```python
from build123d import *

# Parameters (mm, degrees)
SKETCH1_W           = 147.32
SKETCH1_H           = 63.5
BOSS_EXTRUDE3_DEPTH = 5.08
FILLET4_R           = 12.7
SKETCH4_W           = 121.92
SKETCH4_H           = 63.5
SKETCH4_W_2         = 116.84
SKETCH4_H_2         = 58.42
BOSS_EXTRUDE4_DEPTH = 30.48
SKETCH9_W           = 10.16
SKETCH9_H           = 10.16
BOSS_EXTRUDE5_DEPTH = 5.08
FILLET9_R           = 5.08
SKETCH10_R          = 3.175
CUT_EXTRUDE7_DEPTH  = 163.421034352
FILLET11_R          = 5.08
FILLET12_R          = 7.62
CUT_EXTRUDE8_REACH  = 166.317
SKETCH12_W          = 15.24
SKETCH12_H          = 10.16
FILLET13_R          = 2.54
SKETCH13_W          = 7.62
SKETCH13_H          = 10.16
CUT_EXTRUDE9_DEPTH  = 165.316602935
FILLET14_R          = 2.032
SKETCH11_R          = 3.175
SKETCH11_R_2        = 1.27
BOSS_EXTRUDE7_DEPTH = 5.08
SKETCH15_R          = 1.27
CUT_EXTRUDE10_DEPTH = 2.54
BOSS_EXTRUDE9_START = -2.54
SKETCH16_R          = 3.175
BOSS_EXTRUDE9_DEPTH = 2.54


with BuildPart() as part:
    # Sketch1 → Boss-Extrude3 (new body)
    with BuildSketch(Plane(origin=(0, 0, 0), x_dir=(1, 0, 0), z_dir=(0, 1, 0))):
        with Locations((73.66, 31.75)):
            Rectangle(SKETCH1_W, SKETCH1_H)
    extrude(amount=BOSS_EXTRUDE3_DEPTH)

    # Fillet4
    fillet4_edges = [part.edges().sort_by_distance(p)[0] for p in [
        (0, 2.54, -63.5),
        (147.32, 2.54, -63.5),
        (147.32, 2.54, 0),
        (0, 2.54, 0),
    ]]
    fillet(fillet4_edges, radius=FILLET4_R)

    # Sketch4 → Boss-Extrude4 (add)
    with BuildSketch(Plane(origin=(0, 5.08, 0), x_dir=(1, 0, 0), z_dir=(0, 1, 0))):
        with Locations((73.66, 31.75)):
            Rectangle(SKETCH4_W, SKETCH4_H)
        with Locations((73.66, 31.75)):
            Rectangle(SKETCH4_W_2, SKETCH4_H_2, mode=Mode.SUBTRACT)
    extrude(amount=BOSS_EXTRUDE4_DEPTH)

    # Sketch9 → Boss-Extrude5 (add)
    with BuildSketch(Plane(origin=(0, 5.08, 0), x_dir=(1, 0, 0), z_dir=(0, 1, 0))):
        with Locations((20.32, 55.88)):
            Rectangle(SKETCH9_W, SKETCH9_H)
        with Locations((127, 55.88)):
            Rectangle(SKETCH9_W, SKETCH9_H)
        with Locations((127, 7.62)):
            Rectangle(SKETCH9_W, SKETCH9_H)
        with Locations((20.32, 7.62)):
            Rectangle(SKETCH9_W, SKETCH9_H)
    extrude(amount=BOSS_EXTRUDE5_DEPTH)

    # Fillet9
    fillet9_edges = [part.edges().sort_by_distance(p)[0] for p in [
        (25.4, 7.62, -12.7),
        (25.4, 7.62, -50.8),
        (121.92, 7.62, -50.8),
        (121.92, 7.62, -12.7),
    ]]
    fillet(fillet9_edges, radius=FILLET9_R)

    # Sketch10 → Cut-Extrude7 (cut, through all)
    with BuildSketch(Plane(origin=(0, 10.16, 0), x_dir=(1, 0, 0), z_dir=(0, 1, 0))):
        with Locations(Location((20.32, 55.88, 0), (0, 0, 270))):
            Circle(SKETCH10_R)
        with Locations(Location((127, 55.88, 0), (0, 0, 270))):
            Circle(SKETCH10_R)
        with Locations(Location((20.32, 7.62, 0), (0, 0, 270))):
            Circle(SKETCH10_R)
        with Locations(Location((127, 7.62, 0), (0, 0, 270))):
            Circle(SKETCH10_R)
    extrude(amount=-CUT_EXTRUDE7_DEPTH, mode=Mode.SUBTRACT)

    # Fillet11
    fillet11_edges = [part.edges().sort_by_distance(p)[0] for p in [
        (15.24, 22.86, -2.54),
        (132.08, 22.86, -2.54),
        (132.08, 22.86, -60.96),
        (15.24, 22.86, -60.96),
    ]]
    fillet(fillet11_edges, radius=FILLET11_R)

    # Fillet12
    fillet12_edges = [part.edges().sort_by_distance(p)[0] for p in [
        (12.7, 20.32, -63.5),
        (12.7, 20.32, 0),
        (134.62, 20.32, 0),
        (134.62, 20.32, -63.5),
    ]]
    fillet(fillet12_edges, radius=FILLET12_R)

    # Sketch12 → Cut-Extrude8 (cut, up to next)
    with BuildSketch(Plane.XY, mode=Mode.PRIVATE) as cut_extrude8_sk1:
        with Locations((105.41, 24.257)):
            Rectangle(SKETCH12_W, SKETCH12_H)
    cut_extrude8_tool1 = extrude(cut_extrude8_sk1.sketch, amount=-CUT_EXTRUDE8_REACH, mode=Mode.PRIVATE) & part.part
    add(cut_extrude8_tool1.solids().sort_by_distance((105.41, 24.257, 0))[0], mode=Mode.SUBTRACT)

    # Fillet13
    fillet13_edges = [part.edges().sort_by_distance(p)[0] for p in [
        (97.79, 19.177, -1.27),
        (97.79, 29.337, -1.27),
        (113.03, 29.337, -1.27),
        (113.03, 19.177, -1.27),
    ]]
    fillet(fillet13_edges, radius=FILLET13_R)

    # Sketch13 → Cut-Extrude9 (cut, through all)
    with BuildSketch(Plane.XY):
        with Locations((30.48, 15.24)):
            Rectangle(SKETCH13_W, SKETCH13_H)
        with Locations((53.34, 15.24)):
            Rectangle(SKETCH13_W, SKETCH13_H)
    extrude(amount=-CUT_EXTRUDE9_DEPTH, mode=Mode.SUBTRACT)

    # Fillet14
    fillet14_edges = [part.edges().sort_by_distance(p)[0] for p in [
        (26.67, 10.16, -1.27),
        (26.67, 20.32, -1.27),
        (34.29, 20.32, -1.27),
        (34.29, 10.16, -1.27),
        (26.67, 10.16, -62.23),
        (26.67, 20.32, -62.23),
        (34.29, 20.32, -62.23),
        (34.29, 10.16, -62.23),
        (49.53, 10.16, -1.27),
        (49.53, 20.32, -1.27),
        (57.15, 20.32, -1.27),
        (57.15, 10.16, -1.27),
        (49.53, 10.16, -62.23),
        (49.53, 20.32, -62.23),
        (57.15, 20.32, -62.23),
        (57.15, 10.16, -62.23),
    ]]
    fillet(fillet14_edges, radius=FILLET14_R)

    # Sketch11 → Boss-Extrude7 (add)
    # profile 1 of 4: a face of its own
    with BuildSketch(Plane(origin=(0, 10.16, 0), x_dir=(1, 0, 0), z_dir=(0, 1, 0))):
        with Locations(Location((20.32, 55.88, 0), (0, 0, 270))):
            Circle(SKETCH11_R)
        with Locations(Location((20.32, 55.88, 0), (0, 0, 270))):
            Circle(SKETCH11_R_2, mode=Mode.SUBTRACT)
    # profile 2 of 4: a face of its own
    with BuildSketch(Plane(origin=(0, 10.16, 0), x_dir=(1, 0, 0), z_dir=(0, 1, 0))):
        with Locations(Location((127, 55.88, 0), (0, 0, 270))):
            Circle(SKETCH11_R)
        with Locations(Location((127, 55.88, 0), (0, 0, 270))):
            Circle(SKETCH11_R_2, mode=Mode.SUBTRACT)
    # profile 3 of 4: a face of its own
    with BuildSketch(Plane(origin=(0, 10.16, 0), x_dir=(1, 0, 0), z_dir=(0, 1, 0))):
        with Locations(Location((20.32, 7.62, 0), (0, 0, 270))):
            Circle(SKETCH11_R)
        with Locations(Location((20.32, 7.62, 0), (0, 0, 270))):
            Circle(SKETCH11_R_2, mode=Mode.SUBTRACT)
    # profile 4 of 4: a face of its own
    with BuildSketch(Plane(origin=(0, 10.16, 0), x_dir=(1, 0, 0), z_dir=(0, 1, 0))):
        with Locations(Location((127, 7.62, 0), (0, 0, 270))):
            Circle(SKETCH11_R)
        with Locations(Location((127, 7.62, 0), (0, 0, 270))):
            Circle(SKETCH11_R_2, mode=Mode.SUBTRACT)
    extrude(amount=-BOSS_EXTRUDE7_DEPTH)

    # Sketch15 → Cut-Extrude10 (cut)
    with BuildSketch(Plane(origin=(0, 5.08, 0), x_dir=(1, 0, 0), z_dir=(0, 1, 0))):
        with Locations(Location((6.35, 50.8, 0), (0, 0, 270))):
            Circle(SKETCH15_R)
        with Locations(Location((6.35, 12.7, 0), (0, 0, 270))):
            Circle(SKETCH15_R)
        with Locations(Location((140.97, 12.7, 0), (0, 0, 90))):
            Circle(SKETCH15_R)
        with Locations(Location((140.97, 50.8, 0), (0, 0, 90))):
            Circle(SKETCH15_R)
    extrude(amount=-CUT_EXTRUDE10_DEPTH, mode=Mode.SUBTRACT)

    # Sketch16 → Boss-Extrude9 (add)
    with BuildSketch(Plane.XZ.offset(BOSS_EXTRUDE9_START)):
        with Locations(Location((20.32, -7.62, 0), (0, 0, 90))):
            Circle(SKETCH16_R)
        with Locations(Location((127, -7.62, 0), (0, 0, 90))):
            Circle(SKETCH16_R)
        with Locations(Location((20.32, -55.88, 0), (0, 0, 90))):
            Circle(SKETCH16_R)
        with Locations(Location((127, -55.88, 0), (0, 0, 90))):
            Circle(SKETCH16_R)
    extrude(amount=BOSS_EXTRUDE9_DEPTH)


solid = part.part
```
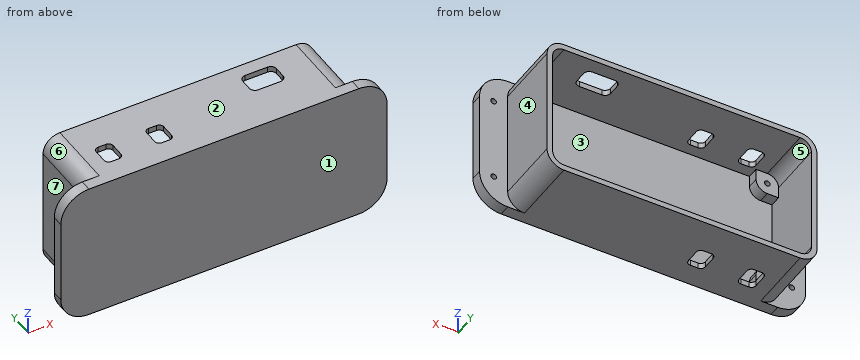
Here's how the part is built. I have some questions about the finished solid (model axes, mm). Face numbers are marked on the shaded views. A direction names the side the tool comes from. Round coordinates to 2 decimals unless told otherwise and drop trailing zeros. Write each loop counter-clockwise with the first axis right and the second up, starting at its lowest first coordinate (ties: lowest second). Pieces come first, ordered by that corner, then holes. Notation, with made-up numbers: M 38.5,45 L 48.5,45 A30 ccw 48.5,78 Z; hole C 50.5,3.25 d1. An arc over 180 degrees is marked long. Answer as CSV lines item,"result". Start each with the question number.
1. Suppose I cut it at A-A on z = -27. Write out the boundary of the cut face in (x, y).
2. I need wall thicknesses on probe 1 along X at (y, z) = (8.9, -55.88); probe 2 along Z at (x, y) = (20, 4); probe 3 along Z at (x, y) = (127, 3) (3 decimals). Which ranges of each line are inside material? Lowest first, please.
3. Suppose I cut it at B-B on x = 89.5. Write out the boundary of the cut face in (y, z).
4. On a 3-axis mill with a long thin cutter (end or side, diameter ignored), from which of +Z, -Z, +X, -X, +Y, -Y can I reach the whole of each face in a straight line? I mean the marked faces 4, 5, 6 and 7. Say none if no direction works.
5. I'm going to push flat-ended pins straight in: pin 1 Ø3 at (y, z) = (15.5, -61.5) entering from +X; pin 2 Ø5 at (y, z) = (27, -7) entering from -X; pin 3 Ø3 at (y, z) = (15, -1.5) entering from -X. Where does each tip first touch, or does it pass through?
6. Thinking about a two-plate mould opening in Z: for the marked faces 1, 2 and 3, which applies, released by +Z, released by -Z, zero draft, split by the parting line, or undercut?
Check result:
1,outline,"M 0,0 L 147.32,0 L 147.32,5.08 L 134.62,5.08 L 134.62,35.56 L 132.08,35.56 L 132.08,5.08 L 15.24,5.08 L 15.24,35.56 L 12.7,35.56 L 12.7,5.08 L 0,5.08 Z"
2,probe 1,"x = 12.7 to 19.05, 21.59 to 25.4, 121.92 to 125.73, 128.27 to 134.62"
2,probe 2,"z = -63.5 to -59.04, -52.72 to -10.78, -4.46 to 0"
2,probe 3,"z = -63.5 to -59.055, -52.705 to -10.795, -4.445 to 0"
3,outline,"M 0,-63.5 L 35.56,-63.5 L 35.56,-60.96 L 5.08,-60.96 L 5.08,-2.54 L 35.56,-2.54 L 35.56,0 L 0,0 Z"
4,face 4,"+Z, -Z, +X, +Y"
4,face 5,"+Y"
4,face 6,"+Z, -X, +Y"
4,face 7,"+Z, -Z, -X, +Y"
5,pin 1,"stops at x = 133.41"
5,pin 2,"stops at x = 12.7"
5,pin 3,"stops at x = 14.26"
6,face 1,"zero draft"
6,face 2,"released by +Z"
6,face 3,"undercut"
